Part model, mm, in its own coordinate system. Face numbers are marked on the shaded views. A direction names the side the tool comes from. Round coordinates to 2 decimals unless told otherwise and drop trailing zeros. Loops run counter-clockwise (first coordinate to the right, second up) from the corner with the lowest first, then second, coordinate; pieces in that order, holes last.
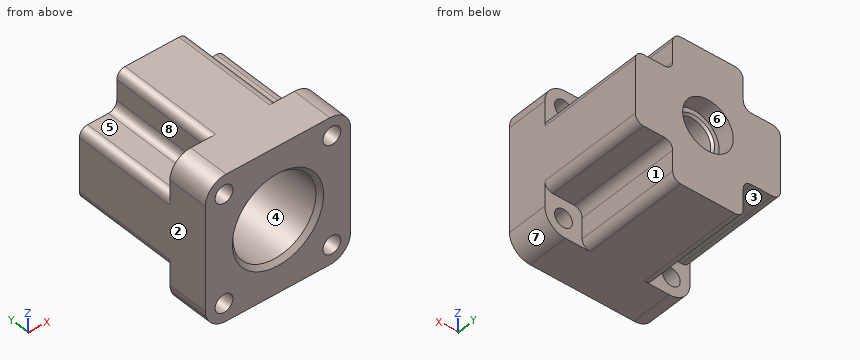
from build123d import *
from build123d.topology import SkipClean

# Parameters (mm, degrees)
SKETCH_1_W          = 35
SKETCH_1_H          = 35
SKETCH_1_R          = 4.5
SKETCH_1_R_2        = 2.15
EXTRUDE_1_DEPTH     = 25
FILLET_1_R          = 5
SKETCH_3_R          = 6.1
CUT_EXTRUDE_1_DEPTH = 4
SKETCH_4_R          = 6.1
CUT_EXTRUDE_2_DEPTH = 4
SKETCH_6_R          = 10
CUT_EXTRUDE_3_DEPTH = 9
EXTRUDE_START       = 10.6
SKETCH_7_R          = 2.15
SKETCH_7_R_2        = 10
EXTRUDE_2_DEPTH     = 10.6
SKETCH_8_W          = 9
SKETCH_8_H          = 9
CUT_EXTRUDE_4_DEPTH = 25.6
FILLET_2_R          = 2
CHAMFER_1_SIZE      = 1
CHAMFER_2_SIZE      = 0.5


with BuildPart() as part:
    # 草图1 → 凸台-拉伸1 (new body)
    with BuildSketch(Plane(origin=(0, 0, 0), x_dir=(1, 0, 0), z_dir=(0, 1, 0))):
        Rectangle(SKETCH_1_W, SKETCH_1_H)
        with Locations(Location((0, 0, 0), (0, 0, 270))):
            Circle(SKETCH_1_R, mode=Mode.SUBTRACT)
        with Locations(Location((13, 13, 0), (0, 0, 270))):
            Circle(SKETCH_1_R_2, mode=Mode.SUBTRACT)
        with Locations(Location((13, -13, 0), (0, 0, 270))):
            Circle(SKETCH_1_R_2, mode=Mode.SUBTRACT)
        with Locations(Location((-13, -13, 0), (0, 0, 270))):
            Circle(SKETCH_1_R_2, mode=Mode.SUBTRACT)
        with Locations(Location((-13, 13, 0), (0, 0, 270))):
            Circle(SKETCH_1_R_2, mode=Mode.SUBTRACT)
    extrude(amount=EXTRUDE_1_DEPTH)

    # 圆角1
    fillet_1_edges = [part.edges().sort_by_distance(p)[0] for p in [
        (17.5, 12.5, 17.5),
        (-17.5, 12.5, 17.5),
        (-17.5, 12.5, -17.5),
        (17.5, 12.5, -17.5),
    ]]
    fillet(fillet_1_edges, radius=FILLET_1_R)

    # 草图3 → 切除-拉伸1 (cut)
    with BuildSketch(Plane(origin=(0, 25, 0), x_dir=(1, 0, 0), z_dir=(0, 1, 0))):
        with Locations(Location((0, 0, 0), (0, 0, 270))):
            Circle(SKETCH_3_R)
    extrude(amount=-CUT_EXTRUDE_1_DEPTH, mode=Mode.SUBTRACT)

    # 草图4 → 切除-拉伸2 (cut)
    with BuildSketch(Plane(origin=(0, 13, 0), x_dir=(1, 0, 0), z_dir=(0, 1, 0))):
        with Locations(Location((0, 0, 0), (0, 0, 270))):
            Circle(SKETCH_4_R)
    extrude(amount=-CUT_EXTRUDE_2_DEPTH, mode=Mode.SUBTRACT)

    # 草图6 → 切除-拉伸3 (cut)
    with BuildSketch(Plane.XZ):
        with Locations(Location((0, 0, 0), (0, 0, 270))):
            Circle(SKETCH_6_R)
    extrude(amount=-CUT_EXTRUDE_3_DEPTH, mode=Mode.SUBTRACT)

    # 草图7 → 凸台-拉伸2 (add)
    with SkipClean():  # the faces are left unmerged after this step: merging them gives an invalid solid
        with BuildSketch(Plane.XZ.offset(EXTRUDE_START)):
            with BuildLine():
                Line((-12.5, -17.5), (12.5, -17.5))
                ThreePointArc((12.5, -17.5), (16.035533906, -16.035533906), (17.5, -12.5))
                Line((17.5, -12.5), (17.5, 12.5))
                ThreePointArc((17.5, 12.5), (16.035533906, 16.035533906), (12.5, 17.5))
                Line((12.5, 17.5), (-12.5, 17.5))
                ThreePointArc((-12.5, 17.5), (-16.035533906, 16.035533906), (-17.5, 12.5))
                Line((-17.5, 12.5), (-17.5, -12.5))
                ThreePointArc((-17.5, -12.5), (-16.035533906, -16.035533906), (-12.5, -17.5))
            make_face()
            with Locations(Location((-13, -13, 0), (0, 0, 270))):
                Circle(SKETCH_7_R, mode=Mode.SUBTRACT)
            with Locations(Location((-13, 13, 0), (0, 0, 270))):
                Circle(SKETCH_7_R, mode=Mode.SUBTRACT)
            with Locations(Location((0, 0, 0), (0, 0, 270))):
                Circle(SKETCH_7_R_2, mode=Mode.SUBTRACT)
            with Locations(Location((13, -13, 0), (0, 0, 270))):
                Circle(SKETCH_7_R, mode=Mode.SUBTRACT)
            with Locations(Location((13, 13, 0), (0, 0, 270))):
                Circle(SKETCH_7_R, mode=Mode.SUBTRACT)
        extrude(amount=-EXTRUDE_2_DEPTH)

    # 草图8 → 切除-拉伸4 (cut)
    with BuildSketch(Plane(origin=(0, 25, 0), x_dir=(1, 0, 0), z_dir=(0, 1, 0))):
        with Locations((-13, 13)):
            Rectangle(SKETCH_8_W, SKETCH_8_H)
        with Locations((13, 13)):
            Rectangle(SKETCH_8_W, SKETCH_8_H)
        with Locations((13, -13)):
            Rectangle(SKETCH_8_W, SKETCH_8_H)
        with Locations((-13, -13)):
            Rectangle(SKETCH_8_W, SKETCH_8_H)
    extrude(amount=-CUT_EXTRUDE_4_DEPTH, mode=Mode.SUBTRACT)

    # 圆角2
    fillet_2_edges = [part.edges().sort_by_distance(p)[0] for p in [
        (-17.5, 12.2, 8.5),
        (-8.5, 12.2, 8.5),
        (-8.5, 12.2, 17.5),
        (8.5, 12.2, 17.5),
        (8.5, 12.2, 8.5),
        (17.5, 12.2, 8.5),
        (17.5, 12.2, -8.5),
        (8.5, 12.2, -8.5),
        (8.5, 12.2, -17.5),
        (-17.5, 12.2, -8.5),
        (-8.5, 12.2, -17.5),
        (-8.5, 12.2, -8.5),
    ]]
    fillet(fillet_2_edges, radius=FILLET_2_R)

    # 倒角1
    chamfer_1_edges = [part.edges().sort_by_distance(p)[0] for p in [
        (0, -10.6, 10),
    ]]
    chamfer(chamfer_1_edges, length=CHAMFER_1_SIZE)

    # 倒角2
    chamfer_2_edges = [part.edges().sort_by_distance(p)[0] for p in [
        (0, 21, -4.5),
        (0, 13, -4.5),
    ]]
    chamfer(chamfer_2_edges, length=CHAMFER_2_SIZE)


solid = part.part
1) Wall check: line 1 along X through (y, z) = (-3, 13); line 2 along Y through (x, z) = (-15, -14); line 3 along Z through (x, y) = (4, 17). Give the ranges that are in metal, low to high.
Values:
line 1: x = -17.47 to -15.15, -10.85 to 10.85, 15.15 to 17.47
line 2: y = -10.6 to -0.6
line 3: z = -17.5 to -2.06, 2.06 to 17.5
2) Slice it at C-C, the plane z = 0. Give the cut face in (x, y).
Values:
outline: (-17.5, -10.6) - (-11, -10.6) - (-10, -9.6) - (-10, 9) - (-6.1, 9) - (-6.1, 13) - (-5, 13) - (-4.5, 13.5) - (-4.5, 20.5) - (-5, 21) - (-6.1, 21) - (-6.1, 25) - (-17.5, 25) - close; (4.5, 13.5) - (5, 13) - (6.1, 13) - (6.1, 9) - (10, 9) - (10, -9.6) - (11, -10.6) - (17.5, -10.6) - (17.5, 25) - (6.1, 25) - (6.1, 21) - (5, 21) - (4.5, 20.5) - close
3) Slice it at A-A, the plane x = 0. Give the cut face in (y, z).
Values:
outline: (-10.6, -17.5) - (25, -17.5) - (25, -6.1) - (21, -6.1) - (21, -5) - (20.5, -4.5) - (13.5, -4.5) - (13, -5) - (13, -6.1) - (9, -6.1) - (9, -10) - (-9.6, -10) - (-10.6, -11) - close; (-10.6, 11) - (-9.6, 10) - (9, 10) - (9, 6.1) - (13, 6.1) - (13, 5) - (13.5, 4.5) - (20.5, 4.5) - (21, 5) - (21, 6.1) - (25, 6.1) - (25, 17.5) - (-10.6, 17.5) - close
4) Tool access for the marked faces 1, 2, 3, 4 and 5: list every direction of +Z, -Z, +X, -X, +Y, -Y with a clear straight run to the whole face (end or side of a thin tool).
Values:
face 1: -Z, +X, +Y
face 2: +Z, -Z, -X, +Y, -Y
face 3: -Z, -X, +Y
face 4: -Y
face 5: +Z, -X, +Y
5) Slice it at D-D, the plane x = -13. Give the cut face in (y, z), then the cut area to 3 significant figures.
Values:
outline: (-10.6, -17.47) - (-0.6, -17.47) - (-0.6, -15.15) - (-10.6, -15.15) - close; (-10.6, -10.85) - (-0.6, -10.85) - (-0.6, -8.5) - (25, -8.5) - (25, 8.5) - (-0.6, 8.5) - (-0.6, 10.85) - (-10.6, 10.85) - close; (-10.6, 15.15) - (-0.6, 15.15) - (-0.6, 17.47) - (-10.6, 17.47) - close
area: 699 mm2
6) Slice it at B-B, the plane y = 5.5. Give the cut face in (x, z).
Values:
outline: (-17.5, -6.5) arc R2 ccw to (-15.5, -8.5) - (-10.5, -8.5) arc R2 cw to (-8.5, -10.5) - (-8.5, -15.5) arc R2 ccw to (-6.5, -17.5) - (6.5, -17.5) arc R2 ccw to (8.5, -15.5) - (8.5, -10.5) arc R2 cw to (10.5, -8.5) - (15.5, -8.5) arc R2 ccw to (17.5, -6.5) - (17.5, 6.5) arc R2 ccw to (15.5, 8.5) - (10.5, 8.5) arc R2 cw to (8.5, 10.5) - (8.5, 15.5) arc R2 ccw to (6.5, 17.5) - (-6.5, 17.5) arc R2 ccw to (-8.5, 15.5) - (-8.5, 10.5) arc R2 cw to (-10.5, 8.5) - (-15.5, 8.5) arc R2 ccw to (-17.5, 6.5) - close; hole circle Ø20 at (0, 0)
7) Drop flat-ended pins along their axis: pin 1 Ø9 at (x, z) = (14, 10.5) entering from +Y; pin 2 Ø6 at (x, z) = (1.5, -2.5) entering from -Y; pin 3 Ø8 at (x, z) = (-1, -6) entering from -Y; pin 4 Ø5.5 at (y, z) = (11, 14) entering from -X. Give the stop position or say it passes through.
Values:
pin 1: stops at y = 25
pin 2: stops at y = 13
pin 3: stops at y = -9.68
pin 4: stops at x = -8.5
8) Mould opens along X. For the marked faces 6, 7 and 8 say: released by +X, released by -X, zero draft, split by the parting line, or undercut.
Values:
face 6: undercut
face 7: released by +X
face 8: released by -X
